from build123d import *

# Parameters (mm, degrees)
SKETCH3_W                          = 158.75
SKETCH3_H                          = 107.95
BASE_EXTRUDE_DEPTH                 = 4.572
SKETCH4_W                          = 20.6375
SKETCH4_H                          = 1.778
SKETCH4_W_2                        = 139.7
SKETCH4_H_2                        = 38.1
VELCRO_SLITS_DEPTH                 = 193.030383492
SKETCH6_W                          = 2.286
SKETCH6_H                          = 12.7
SKETCH6_W_2                        = 12.7
SKETCH6_H_2                        = 3.81
SKETCH6_H_3                        = 6.858
POSITION_GUIDES_DEPTH              = 5.08
FILLET1_R                          = 1.27
SKETCH7_R                          = 1.905
SKETCH7_W                          = 12.7
SKETCH7_H                          = 38.1
RIGHT_SCREW_HOLE_AND_SUPPORT_DEPTH = 4.572
SKETCH10_R                         = 1.905
LEFT_SCREW_HOLE_DEPTH              = 193.043149839
FILLET2_R                          = 5.08
SKETCH11_R                         = 3.048
SCREWHEAD_CUTOUTS_DEPTH            = 3.81
SKETCH5_W                          = 20.6375
SKETCH5_H                          = 1.524
CUT_EXTRUDE1_DEPTH                 = 193.21843331


with BuildPart() as part:
    # Sketch3 → Base Extrude (new body)
    with BuildSketch(Plane(origin=(0, 0, 0), x_dir=(1, 0, 0), z_dir=(0, 1, 0))):
        with Locations((79.375, 53.975)):
            Rectangle(SKETCH3_W, SKETCH3_H)
    extrude(amount=BASE_EXTRUDE_DEPTH)

    # Sketch4 → Velcro slits (cut, through all)
    with BuildSketch(Plane(origin=(0, 4.572, 0), x_dir=(1, 0, 0), z_dir=(0, 1, 0))):
        with Locations((79.375, 104.521)):
            Rectangle(SKETCH4_W, SKETCH4_H)
        with Locations((79.375, 55.753)):
            Rectangle(SKETCH4_W, SKETCH4_H)
        with Locations((79.375, 52.197)):
            Rectangle(SKETCH4_W, SKETCH4_H)
        with Locations((79.375, 3.429)):
            Rectangle(SKETCH4_W, SKETCH4_H)
        with Locations((79.375, 27.813)):
            Rectangle(SKETCH4_W_2, SKETCH4_H_2)
        with Locations((79.375, 80.137)):
            Rectangle(SKETCH4_W_2, SKETCH4_H_2)
    extrude(amount=-VELCRO_SLITS_DEPTH, mode=Mode.SUBTRACT)

    # Sketch6 → Position Guides (add)
    with BuildSketch(Plane(origin=(0, 4.572, 0), x_dir=(1, 0, 0), z_dir=(0, 1, 0))):
        Polygon((2.286, 16.51), (2.286, 3.81), (25.4, 3.81), (25.4, 0), (0, 0), (0, 16.51), align=None)
        Polygon((2.286, 41.275), (2.286, 50.546), (25.4, 50.546), (25.4, 57.404), (2.286, 57.404), (2.286, 66.675), (0, 66.675), (0, 41.275), align=None)
        Polygon((0, 91.44), (2.286, 91.44), (2.286, 104.14), (25.4, 104.14), (25.4, 107.95), (0, 107.95), align=None)
        with Locations((157.607, 80.137)):
            Rectangle(SKETCH6_W, SKETCH6_H)
        with Locations((157.607, 27.813)):
            Rectangle(SKETCH6_W, SKETCH6_H)
        with Locations((127, 106.045)):
            Rectangle(SKETCH6_W_2, SKETCH6_H_2)
        with Locations((127, 53.975)):
            Rectangle(SKETCH6_W_2, SKETCH6_H_3)
        with Locations((127, 1.905)):
            Rectangle(SKETCH6_W_2, SKETCH6_H_2)
    extrude(amount=POSITION_GUIDES_DEPTH)

    # Fillet1
    fillet1_edges = [part.edges().sort_by_distance(p)[0] for p in [
        (2.286, 7.112, -16.51),
        (25.4, 7.112, -3.81),
        (2.286, 7.112, -3.81),
        (2.286, 7.112, -41.275),
        (2.286, 7.112, -50.546),
        (25.4, 7.112, -50.546),
        (25.4, 7.112, -57.404),
        (2.286, 7.112, -57.404),
        (2.286, 7.112, -66.675),
        (2.286, 7.112, -91.44),
        (2.286, 7.112, -104.14),
        (25.4, 7.112, -104.14),
        (156.464, 7.112, -86.487),
        (156.464, 7.112, -73.787),
        (156.464, 7.112, -34.163),
        (156.464, 7.112, -21.463),
        (120.65, 7.112, -57.404),
        (120.65, 7.112, -50.546),
        (133.35, 7.112, -50.546),
        (133.35, 7.112, -57.404),
        (133.35, 7.112, -104.14),
        (120.65, 7.112, -104.14),
        (133.35, 7.112, -3.81),
        (120.65, 7.112, -3.81),
    ]]
    fillet(fillet1_edges, radius=FILLET1_R)

    # Sketch7 → Right screw hole and support (add)
    # profile 1 of 2: a face of its own
    with BuildSketch(Plane(origin=(0, 4.572, 0), x_dir=(1, 0, 0), z_dir=(0, 1, 0))):
        with Locations((5.08, 69.85)):
            Circle(SKETCH7_R)
    # profile 2 of 2: a face of its own
    with BuildSketch(Plane(origin=(0, 4.572, 0), x_dir=(1, 0, 0), z_dir=(0, 1, 0))):
        with Locations((65.405, 80.137)):
            Rectangle(SKETCH7_W, SKETCH7_H)
        with Locations(Location((65.405, 73.025, 0), (0, 0, 270))):
            Circle(SKETCH7_R, mode=Mode.SUBTRACT)
    extrude(amount=-RIGHT_SCREW_HOLE_AND_SUPPORT_DEPTH)

    # Sketch10 → Left Screw Hole (cut, through all)
    with BuildSketch(Plane(origin=(0, 4.572, 0), x_dir=(1, 0, 0), z_dir=(0, 1, 0))):
        with Locations(Location((5.08, 69.9135, 0), (0, 0, 270))):
            Circle(SKETCH10_R)
    extrude(amount=-LEFT_SCREW_HOLE_DEPTH, mode=Mode.SUBTRACT)

    # Fillet2
    fillet2_edges = [part.edges().sort_by_distance(p)[0] for p in [
        (59.055, 2.286, -99.187),
        (71.755, 2.286, -99.187),
        (71.755, 2.286, -61.087),
        (59.055, 2.286, -61.087),
        (9.525, 2.286, -8.763),
        (9.525, 2.286, -46.863),
        (149.225, 2.286, -46.863),
        (149.225, 2.286, -8.763),
        (9.525, 2.286, -61.087),
        (9.525, 2.286, -99.187),
        (149.225, 2.286, -99.187),
        (149.225, 2.286, -61.087),
    ]]
    fillet(fillet2_edges, radius=FILLET2_R)

    # Sketch11 → Screwhead cutouts (cut)
    with BuildSketch(Plane(origin=(0, 4.572, 0), x_dir=(1, 0, 0), z_dir=(0, 1, 0))):
        with Locations(Location((5.08, 69.9135, 0), (0, 0, 270))):
            Circle(SKETCH11_R)
        with Locations(Location((65.405, 73.025, 0), (0, 0, 270))):
            Circle(SKETCH11_R)
    extrude(amount=-SCREWHEAD_CUTOUTS_DEPTH, mode=Mode.SUBTRACT)

    # Sketch5 → Cut-Extrude1 (cut, through all)
    with BuildSketch(Plane.XY):
        with Locations((79.375, 0.762)):
            Rectangle(SKETCH5_W, SKETCH5_H)
    extrude(amount=-CUT_EXTRUDE1_DEPTH, mode=Mode.SUBTRACT)


solid = part.part
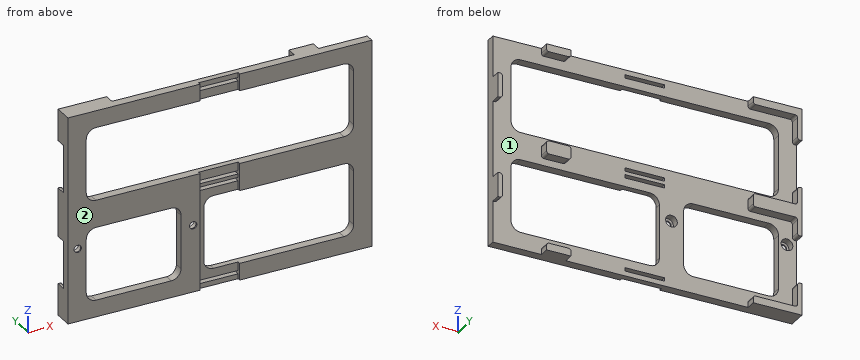
Part model, mm, in its own coordinate system. Face numbers are marked on the shaded views. Give positions to 0.01 mm unless a question says otherwise; leave off trailing zeros. Order: outer loops, then holes, each group sorted by start corner. A loop starts at its lowest first (then second) coordinate and runs counter-clockwise, first axis right, second up. Notation, with made-up numbers: (5.5, -15.75) -> (52.5, -15.75) arc R12 cw to (52.5, 0.25) -> close; hole circle Ø7 at (7, 89.25). An arc over 180 degrees is marked (long way). Use one line per item in the form item = value.
(1) Flat gauge pins, fed straight in: P1, Ø0.8, axis at y = 6.5, z = -1.5, coming from the +X side; P2, Ø0.5, axis at x = 158.5, y = 6, coming from the -Z side; P3, Ø0.5, axis at x = 158.5, y = 6.5, coming from the +Z side; P4, Ø12, axis at x = 80, z = -40.5, coming from the +Y side. Where does each tip first touch, or does it go through?
Solution:
P1 = 133.35
P2 = -86.49
P3 = -21.46
P4 = through
(2) Saw through at C-C (y = 8). Count the separate pieces of the cut face and the enclosed holes in it, then the cut area to 3 significant figures.
Solution:
separate_pieces = 8
enclosed_holes = 0
area = 705 mm²
(3) Drill centre lines: line 1 (X direction, y = 2.5, z = -66.5) (3 decimals); line 2 (Z direction, x = 41, y = 1.5); line 3 (X direction, y = 0.75, z = -88.5) (3 decimals). Where is each one in solid material? Low to high. Write a range as from..to.
Solution:
line_1 = 0..9.525, 59.055..71.755, 149.225..158.75
line_2 = -107.95..-99.19, -61.09..-46.86, -8.76..0
line_3 = 0..9.525, 59.055..69.056, 149.225..158.75
(4) Saw through at B-B (x = 84.5). Write the cut outline in (y, z), then the cut area to 3 significant figures.
Solution:
outline = (1.52, -107.95) -> (4.57, -107.95) -> (4.57, -105.41) -> (1.52, -105.41) -> close; (1.52, -103.63) -> (4.57, -103.63) -> (4.57, -99.19) -> (1.52, -99.19) -> close; (1.52, -61.09) -> (4.57, -61.09) -> (4.57, -56.64) -> (1.52, -56.64) -> close; (1.52, -54.86) -> (4.57, -54.86) -> (4.57, -53.09) -> (1.52, -53.09) -> close; (1.52, -51.31) -> (4.57, -51.31) -> (4.57, -46.86) -> (1.52, -46.86) -> close; (1.52, -8.76) -> (4.57, -8.76) -> (4.57, -4.32) -> (1.52, -4.32) -> close; (1.52, -2.54) -> (4.57, -2.54) -> (4.57, 0) -> (1.52, 0) -> close
area = 75.1 mm²
(5) Pull direction Z, two halves, no side cores. Call the marked faces 1 and 2: +Z half, -Z half, draft (parallel to the pull), parting line (faces both ways), or undercut.
Solution:
face_1 = undercut
face_2 = draft
(6) Saw through at D-D (z = -97). Write the cut outline in (x, y), then the cut area to 3 significant figures.
Solution:
outline = (0, 0) -> (10.43, 0) -> (10.43, 4.57) -> (2.29, 4.57) -> (2.29, 9.65) -> (0, 9.65) -> close; (58.15, 0) -> (69.06, 0) -> (69.06, 1.52) -> (72.66, 1.52) -> (72.66, 4.57) -> (58.15, 4.57) -> close; (148.32, 0) -> (158.75, 0) -> (158.75, 4.57) -> (148.32, 4.57) -> close
area = 168 mm²
(7) Saw through at A-A (z = -26.5). Write the cut outline in (x, y) (3 decimals).
Solution:
outline = (0, 0) -> (9.525, 0) -> (9.525, 4.572) -> (0, 4.572) -> close; (149.225, 0) -> (158.75, 0) -> (158.75, 9.652) -> (156.464, 9.652) -> (156.464, 4.572) -> (149.225, 4.572) -> close
